The drawing under review shows one solid part. Ordinate dimensions are in mm from its lowest x, y, z. A direction names the side the tool comes from. Coordinates: 2 decimals unless noted, no trailing zeros. Loops run counter-clockwise (first coordinate to the right, second up) from the corner with the lowest first, then second, coordinate; pieces in that order, holes last. Notation, with made-up numbers: (16.25, 16.25) - (43.25, 16.25) arc R33 cw to (43.25, 46.25) - close; hole circle Ø6 at (-29.75, 57.5). An arc over 180 degrees is marked (long way). Use one line per item in the form item = value. Start each with the question number.
1. Add section C-C on z = 3. Give the boundary of the cut face in (x, y).
2. Add section A-A on z = 15. Give the boundary of the cut face in (x, y).
3. Machinability: for the marked faces 1 and 2, which of the approach directions +Z, -Z, +X, -X, +Y, -Y give a long, thin tool a straight path to every point of the face, cutting with its end or side? Answer none if there is none.
4. For pin 1 Ø2.5 at (y, z) = (7.5, 15) entering from -X; pin 2 Ø1 at (x, y) = (12, 3.5) entering from +Z; pin 3 Ø8 at (x, z) = (25, 26.5) entering from +Y, all flat-tipped, find the tip position at first contact; note any pin that passes through.
5. To check wall thickness, follow probe 1 along X at (y, z) = (1.3, 15); probe 2 along X at (y, z) = (10.75, 18); probe 3 along Y at (x, z) = (7.75, 24). State the ranges of each line that lie inside material, in increasing order.
6. Draft analysis for pull direction Z (two halves, no side actions). For the marked faces 3, 4 and 5, state which applies: +Z half, -Z half, draft (parallel to the pull), parting line (faces both ways), or undercut.
7. Add section D-D on y = 13.5. Give the boundary of the cut face in (x, z).
8. Add section B-B on x = 27. Give the boundary of the cut face in (y, z).
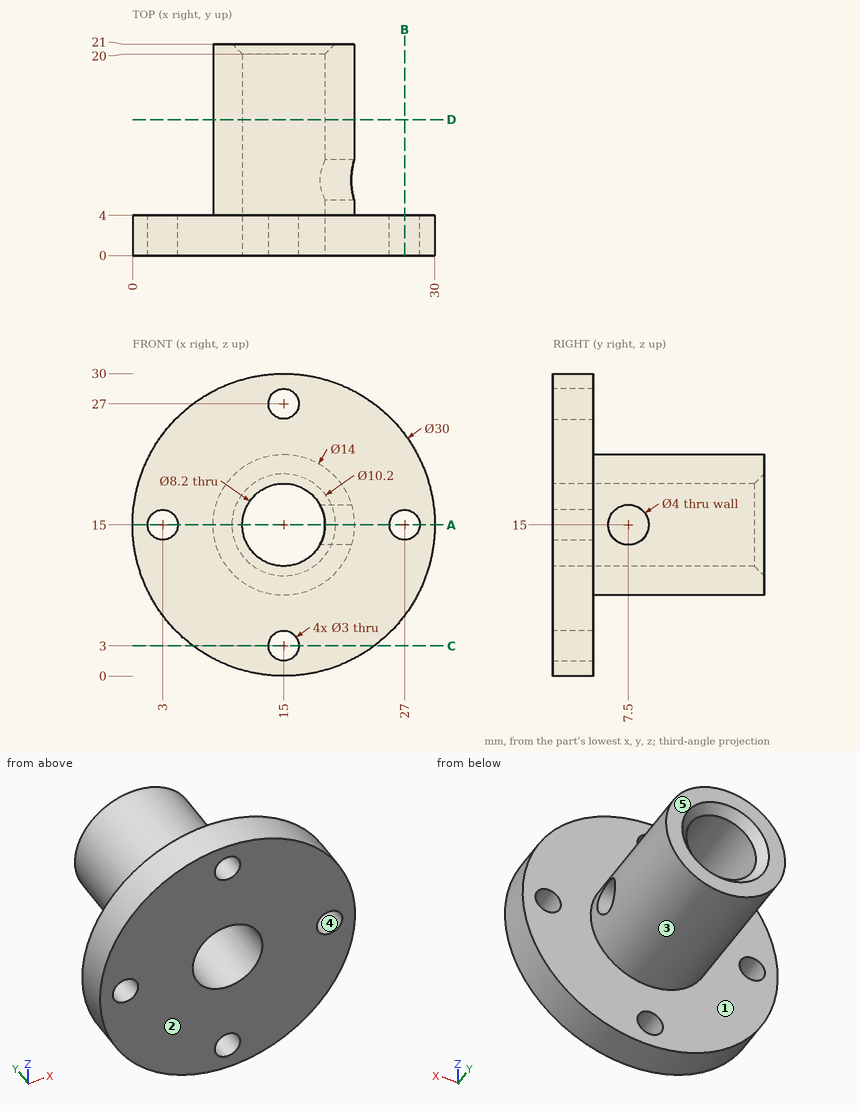
Conclusion:
q1.outline = (6, 0) - (13.5, 0) - (13.5, 4) - (6, 4) - close; (16.5, 0) - (24, 0) - (24, 4) - (16.5, 4) - close
q2.outline = (0, 0) - (1.5, 0) - (1.5, 4) - (0, 4) - close; (4.5, 0) - (10.9, 0) - (10.9, 20) - (9.9, 21) - (8, 21) - (8, 4) - (4.5, 4) - close; (19.1, 0) - (25.5, 0) - (25.5, 4) - (22, 4) - (22, 5.5) - (19.1, 5.5) - close; (19.1, 9.5) - (22, 9.5) - (22, 21) - (20.1, 21) - (19.1, 20) - close; (28.5, 0) - (30, 0) - (30, 4) - (28.5, 4) - close
q3.face_1 = +Y
q3.face_2 = +Z, -Z, +X, -X, -Y
q4.pin_1 = 8
q4.pin_2 = 29.79
q4.pin_3 = 4
q5.probe_1 = 0 to 1.5, 4.5 to 10.9, 19.1 to 25.5, 28.5 to 30
q5.probe_2 = 8.68 to 12.21, 17.79 to 21.32
q5.probe_3 = 0 to 4
q6.face_3 = parting line
q6.face_4 = undercut
q6.face_5 = draft
q7.outline = circle Ø14 at (15, 15); hole circle Ø8.2 at (15, 15)
q8.outline = (0, 6) - (4, 6) - (4, 13.5) - (0, 13.5) - close; (0, 16.5) - (4, 16.5) - (4, 24) - (0, 24) - close
